CAD build for the part. Positions are in the model's coordinates, mm. A direction names the side the tool comes from. Give positions to 0.01 mm unless a question says otherwise; leave off trailing zeros. Write each loop counter-clockwise with the first axis right and the second up, starting at its lowest first coordinate (ties: lowest second). Pieces come first, ordered by that corner, then holes. Notation, with made-up numbers: (55.25, -35.5) - (64.25, -35.5) arc R31 ccw to (64.25, 0.5) - close; hole circle Ø5 at (-7.75, 45.5). An arc over 180 degrees is marked (long way). Answer as a JSON object with one key per item and string values.
Autodesk Inventor part; units mm, degrees
ref_plane "YZ Plane" through (0, 0, 0) normal (1, 0, 0) x (0, 1, 0)
ref_plane "XZ Plane" through (0, 0, 0) normal (0, 1, 0) x (-1, 0, 0)
ref_plane "XY Plane" through (0, 0, 0) normal (0, 0, 1) x (1, 0, 0)
sketch "Sketch1" plane through (0, 0, 0) normal (0, 0, 1) x (1, 0, 0)
  circle A0 centre (0, 0) radius 2.5
  dimension "d0" = 5
extrude "Extrusion1" add sketch "Sketch1" along normal blind 50
sketch "Sketch2" plane through (0, 0, 50) normal (0, 0, 1) x (1, 0, 0)
  circle A0 centre (0, 0) radius 2.5
  circle A1 centre (0, 0) radius 1
  dimension "d3" = 2
extrude "Extrusion2" add sketch "Sketch2" along normal blind 3 contours A1
sketch "Sketch3" plane through (0, 0, 0) normal (0, 0, -1) x (-1, 0, 0)
  circle A0 centre (0, 0) radius 1
  dimension "d6" = 2
extrude "Extrusion3" add sketch "Sketch3" along normal blind 3
properties part number "Bone-5cm"
(1) Saw through at D-D, the plane z = 33.5. Give the cut face in (x, y).
Answer key:
{"outline": "circle Ø5 at (0, 0)"}
(2) Probe L1, parallel to X at y = 0.1, z = 18.5; L2, parallel to Z at x = -2, y = -0.6; L3, parallel to Y at x = 0, z = -1. List the from-to ranges inside material, lowest first. Write a range as [from, to].
Answer key:
{"L1": "x = [-2.5, 2.5]", "L2": "z = [0, 50]", "L3": "y = [-1, 1]"}
(3) 3-axis set-ups, long thin cutter, end or side, ignore diameter. For faces 3 (the face through (0, 0, 53)), 4 (the face through (0, 1, -1)): which of +Z, -Z, +X, -X, +Y, -Y reach the whole face in a straight line?
Answer key:
{"face 3": "+Z, +X, -X, +Y, -Y", "face 4": "-Z"}
(4) Flat gauge pins, fed straight in: P1, Ø1, axis at y = 1, z = 33.5, coming from the -X side; P2, Ø1, axis at y = -1, z = 37.5, coming from the +X side; P3, Ø1, axis at x = 1.5, y = -1.5, coming from the +Z side. Where does each tip first touch, or does it go through?
Answer key:
{"P1": "stops at x = -2.45", "P2": "stops at x = 2.45", "P3": "stops at z = 50"}
(5) Saw through at C-C, the plane z = 50.5. Give the cut face in (x, y), and give its area (3 significant figures).
Answer key:
{"outline": "circle Ø2 at (0, 0)", "area": "3.14 mm²"}
(6) Pull direction Y, two halves, no side cores. Call faces 1 (the face through (0, 1, 51)), 2 (the face through (1, -1, 50)): pulls with the +Y half, pulls with the -Y half, needs draft (parallel to the pull), parting line crosses it, or undercut.
Answer key:
{"face 1": "parting line crosses it", "face 2": "needs draft"}
(7) Saw through at A-A, the plane y = 0. Give the cut face in (x, z), and give its area (3 significant figures).
Answer key:
{"outline": "(-2.5, 0) - (-1, 0) - (-1, -3) - (1, -3) - (1, 0) - (2.5, 0) - (2.5, 50) - (1, 50) - (1, 53) - (-1, 53) - (-1, 50) - (-2.5, 50) - close", "area": "262 mm²"}
